from build123d import *

# Parameters (mm, degrees)
SKETCH_W        = 139.7
SKETCH_H        = 114.3
SKETCH_W_2      = 133.35
SKETCH_H_2      = 107.95
PAD_DEPTH       = 25.4
SKETCH001_W     = 139.7
SKETCH001_H     = 114.3
PAD001_DEPTH    = 3.175
SKETCH002_R     = 5.08
SKETCH002_R_2   = 2.413
PAD002_DEPTH    = 25.4
SKETCH003_W     = 31.75
SKETCH003_H     = 40
PAD003_DEPTH    = 24.5
POCKET_DEPTH    = 139.701
SKETCH007_R     = 4.445
SKETCH007_R_2   = 1.425
PAD006_DEPTH    = 6.35
SKETCH014_R     = 2.2225
POCKET004_DEPTH = 3.176
SKETCH015_W     = 133.35
SKETCH015_H     = 41.402
POCKET005_DEPTH = 6.35
PAD010_DEPTH    = 3.175
PAD011_DEPTH    = 3.175


with BuildPart() as part:
    # Sketch → Pad (new body)
    with BuildSketch(Plane.XY):
        Rectangle(SKETCH_W, SKETCH_H)
        Rectangle(SKETCH_W_2, SKETCH_H_2, mode=Mode.SUBTRACT)
    extrude(amount=PAD_DEPTH)

    # Sketch001 (on Face9 of Pad) → Pad001 (join)
    with BuildSketch(Plane(origin=(0, 0, 0), x_dir=(1, 0, 0), z_dir=(0, 0, -1))):
        Rectangle(SKETCH001_W, SKETCH001_H)
    extrude(amount=PAD001_DEPTH)

    # Sketch002 (on Face15 of Pad001) → Pad002 (join)
    with BuildSketch(Plane.XY):
        with Locations((-64.77, 52.07)):
            Circle(SKETCH002_R)
        with Locations((-64.77, 52.07)):
            Circle(SKETCH002_R_2, mode=Mode.SUBTRACT)
        with Locations((0, 52.07)):
            Circle(SKETCH002_R)
        with Locations((0, 52.07)):
            Circle(SKETCH002_R_2, mode=Mode.SUBTRACT)
        with Locations((64.77, 52.07)):
            Circle(SKETCH002_R)
        with Locations((64.77, 52.07)):
            Circle(SKETCH002_R_2, mode=Mode.SUBTRACT)
        with Locations((64.77, 0)):
            Circle(SKETCH002_R)
        with Locations((64.77, 0)):
            Circle(SKETCH002_R_2, mode=Mode.SUBTRACT)
        with Locations((64.77, -52.07)):
            Circle(SKETCH002_R)
        with Locations((64.77, -52.07)):
            Circle(SKETCH002_R_2, mode=Mode.SUBTRACT)
        with Locations((0, -52.07)):
            Circle(SKETCH002_R)
        with Locations((0, -52.07)):
            Circle(SKETCH002_R_2, mode=Mode.SUBTRACT)
        with Locations((-64.77, -52.07)):
            Circle(SKETCH002_R)
        with Locations((-64.77, -52.07)):
            Circle(SKETCH002_R_2, mode=Mode.SUBTRACT)
        with Locations((-64.77, 0)):
            Circle(SKETCH002_R)
        with Locations((-64.77, 0)):
            Circle(SKETCH002_R_2, mode=Mode.SUBTRACT)
    extrude(amount=PAD002_DEPTH)

    # Sketch003 (on Face43 of Pad002) → Pad003 (join)
    with BuildSketch(Plane.XY):
        with Locations((-53.975, -27.62)):
            Rectangle(SKETCH003_W, SKETCH003_H)
        with Locations((53.975, -27.62)):
            Rectangle(SKETCH003_W, SKETCH003_H)
    extrude(amount=PAD003_DEPTH)

    # Sketch004 (on Face17 of Pad003) → Pocket (cut, through all)
    with BuildSketch(Plane(origin=(-69.85, 0, 0), x_dir=(0, -1, 0), z_dir=(-1, 0, 0))):
        with BuildLine():
            ThreePointArc((18.095, 20.593034), (27.62, 0), (37.145, 20.593034))
            Line((37.145, 26.943034), (37.145, 20.593034))
            Line((18.095, 26.943034), (37.145, 26.943034))
            Line((18.095, 20.593034), (18.095, 26.943034))
        make_face()
    extrude(amount=-POCKET_DEPTH, mode=Mode.SUBTRACT)

    # Sketch007 → Pad006 (join)
    with BuildSketch(Plane(origin=(-34.29, 25.4, 0), x_dir=(1, 0, 0), z_dir=(0, 0, 1))):
        with Locations((12.765624, 13.285831)):
            Circle(SKETCH007_R)
        with Locations((12.765624, 13.285831)):
            Circle(SKETCH007_R_2, mode=Mode.SUBTRACT)
        with Locations((-17.234376, 13.285831)):
            Circle(SKETCH007_R)
        with Locations((-17.234376, 13.285831)):
            Circle(SKETCH007_R_2, mode=Mode.SUBTRACT)
        with Locations((-17.234376, -20.714169)):
            Circle(SKETCH007_R)
        with Locations((-17.234376, -20.714169)):
            Circle(SKETCH007_R_2, mode=Mode.SUBTRACT)
        with Locations((12.765624, -20.714169)):
            Circle(SKETCH007_R)
        with Locations((12.765624, -20.714169)):
            Circle(SKETCH007_R_2, mode=Mode.SUBTRACT)
    extrude(amount=PAD006_DEPTH)

    # Sketch014 (on Face30 of Pad006) → Pocket004 (cut, through all)
    with BuildSketch(Plane.XZ.offset(-53.975)):
        with Locations((-44.45, 14.605)):
            Circle(SKETCH014_R)
        with Locations((-12.7, 5.08)):
            Circle(SKETCH014_R)
        with Locations((12.7, 14.605)):
            Circle(SKETCH014_R)
        with Locations((44.45, 5.08)):
            Circle(SKETCH014_R)
    extrude(amount=-POCKET004_DEPTH, mode=Mode.SUBTRACT)

    # Sketch015 (on Face84 of Pocket004) → Pocket005 (cut)
    with BuildSketch(Plane.XY.offset(24.5)):
        with Locations((0, -27.051)):
            Rectangle(SKETCH015_W, SKETCH015_H)
    extrude(amount=-POCKET005_DEPTH, mode=Mode.SUBTRACT)

    # Sketch016 (on Face15 of Pocket005) → Pad010 (join)
    with BuildSketch(Plane(origin=(-69.85, 0, 0), x_dir=(0, -1, 0), z_dir=(-1, 0, 0))):
        with BuildLine():
            ThreePointArc((18.095, 12.499369), (27.62, 2.97434), (37.145, 12.499369))
            Line((37.145, 20.8996), (37.145, 12.499369))
            ThreePointArc((18.095, 20.8996), (27.62, -0.20066), (37.145, 20.8996))
            Line((18.095, 20.8996), (18.095, 12.499369))
        make_face()
    extrude(amount=-PAD010_DEPTH)

    # Sketch019 (on Face25 of Pocket005) → Pad011 (join)
    with BuildSketch(Plane.YZ.offset(69.85)):
        with BuildLine():
            ThreePointArc((-37.145, 20.8996), (-27.62, -0.20066), (-18.095, 20.8996))
            Line((-18.095, 20.8996), (-18.095, 12.49934))
            ThreePointArc((-37.145, 12.499312), (-27.619986, 2.97434), (-18.095, 12.49934))
            Line((-37.145, 20.8996), (-37.145, 12.499312))
        make_face()
    extrude(amount=-PAD011_DEPTH)


solid = part.part
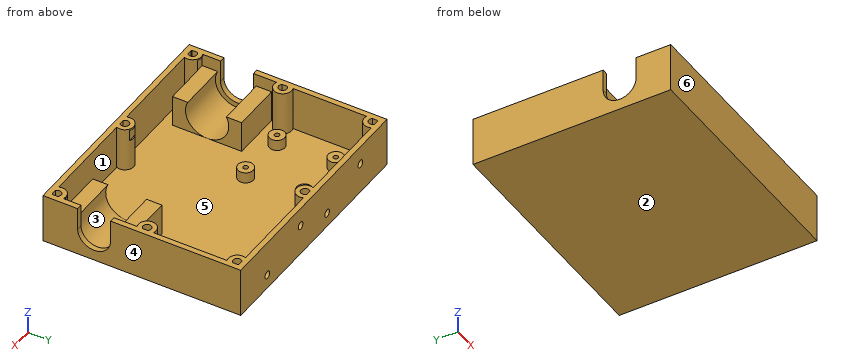
Could you check a few things on this model? Use its own coordinates, in mm. Face numbers are marked on the shaded views. A direction names the side the tool comes from. Round coordinates to 2 decimals unless told otherwise and drop trailing zeros. Loops run counter-clockwise (first coordinate to the right, second up) from the corner with the lowest first, then second, coordinate; pieces in that order, holes last. Notation, with made-up numbers: (64.5, 3.25) -> (86.5, 3.25) arc R16 cw to (86.5, 17.25) -> close; hole circle Ø11 at (65.25, 16.5). An arc over 180 degrees is marked (long way). Use CSV: the item, a comma, the result in double quotes.
(1) If we mould it in two halves opening along X, with no side actions, what happens to the marked faces 4, 5 and 6? For each: +X half, -X half, draft (parallel to the pull), parting line (faces both ways), or undercut.
Return value:
face 4,"+X half"
face 5,"undercut"
face 6,"draft"
(2) Suppose I cut it at B-B on y = -52.07. Write out the boundary of the cut face in (x, z) (3 decimals), plus the area to 3 significant figures.
Return value:
outline,"(-69.85, -3.175) -> (69.85, -3.175) -> (69.85, 25.4) -> (66.675, 25.4) -> (66.675, 0) -> (62.357, 0) -> (62.357, 25.4) -> (59.69, 25.4) -> (59.69, 0) -> (5.08, 0) -> (5.08, 25.4) -> (2.413, 25.4) -> (2.413, 0) -> (-2.413, 0) -> (-2.413, 25.4) -> (-5.08, 25.4) -> (-5.08, 0) -> (-59.69, 0) -> (-59.69, 25.4) -> (-62.357, 25.4) -> (-62.357, 0) -> (-66.675, 0) -> (-66.675, 25.4) -> (-69.85, 25.4) -> close"
area,"876 mm²"
(3) If I drill on probe 1 along Y at (x, z) = (-64.77, 19) (3 decimals); probe 2 along X at (y, z) = (-11.5, 17.5); probe 3 along Z at (x, y) = (44.45, 55.3) (1 decimal), over which ranges is the centre line in solid material (lowest first)? Write a range as [from, to].
Return value:
probe 1,"y = [-57.15, -53.975], [-49.657, -47.752], [-5.08, -2.413], [2.413, 5.08], [46.99, 49.657], [53.975, 57.15]"
probe 2,"x = [-69.85, -38.1], [38.1, 69.85]"
probe 3,"z = [-3.2, 2.9], [7.3, 25.4]"
(4) Will these pins go through, and if not, where does the flat tip stop? pin 1 Ø3 at (x, y) = (-51, -9.5) entering from +Z; pin 2 Ø3 at (x, y) = (-64.77, 0) entering from +Z; pin 3 Ø4.5 at (x, y) = (-51.52, 38.69) entering from +Z.
Return value:
pin 1,"stops at z = 18.15"
pin 2,"stops at z = 0"
pin 3,"stops at z = 6.35"
(5) Suppose I cut it at C-C on z = 20.25. Give the number of separate pieces and of enclosed holes in the cut face, plus the area to 3 significant figures.
Return value:
separate pieces,"2"
enclosed holes,"8"
area,"1,720 mm²"
(6) For the marked faces 1, 2 and 3, which set-ups out of +Z, -Z, +X, -X, +Y, -Y let a thin tool reach every point of the face, with its end or its side?
Return value:
face 1,"+Z"
face 2,"-Z, +X, -X, +Y, -Y"
face 3,"none"
